Job drawing, mm, ordinate dimensions from the low corner. One solid piece. Round coordinates to 2 decimals unless told otherwise and drop trailing zeros. Order: outer loops, then holes, each group sorted by start corner. A loop starts at its lowest first (then second) coordinate and runs counter-clockwise, first axis right, second up. Notation, with made-up numbers: (73, -6.75) -> (104, -6.75) arc R19 ccw to (104, 26.25) -> close; hole circle Ø11 at (-31.75, 38). An arc over 180 degrees is marked (long way). Answer as a JSON object with one key per item and string values. Group by question number.
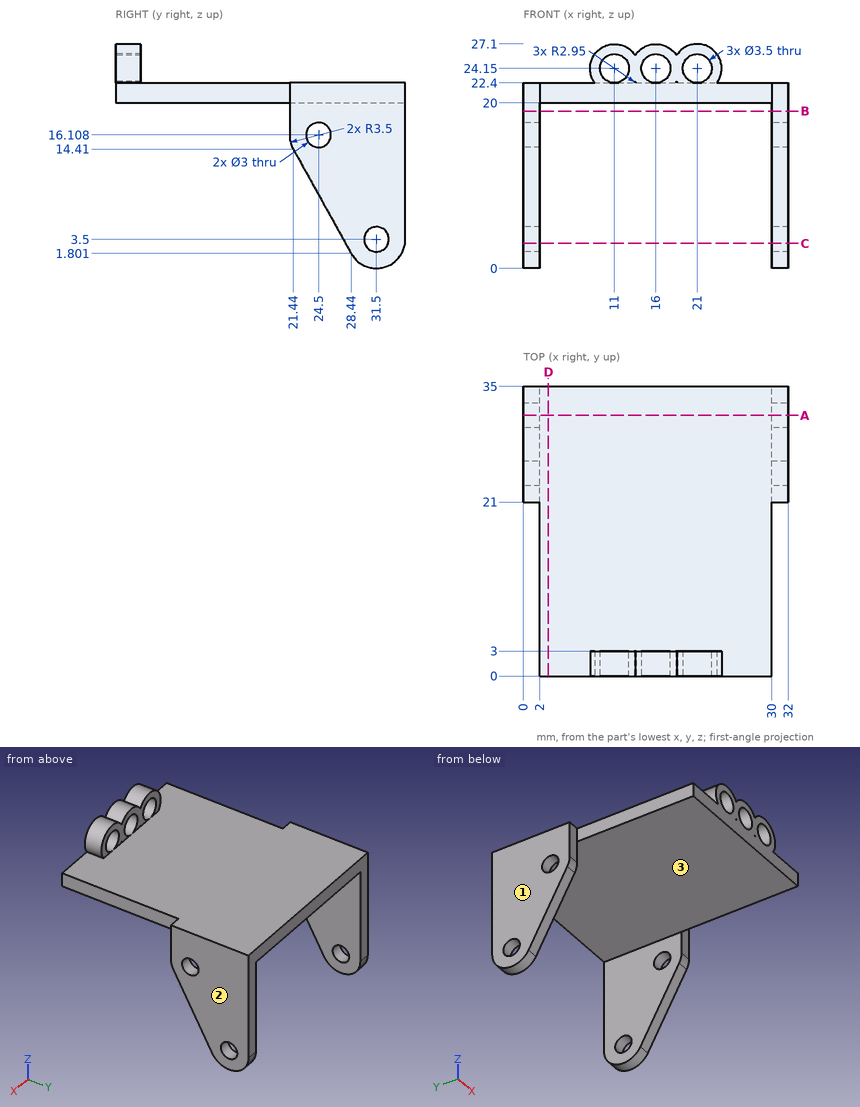
Q1. Band-saw the part on A-A (y = 31.5). List the corners of the cut face in (x, z), plus the area to 3 significant figures.
Q2. Wall check: line 1 (X direction, y = 1.05, z = 24.15); line 2 (Z direction, x = 16, y = 1.5); line 3 (X direction, y = 29.5, z = 8). Give the ranges that are in metal, low to high. Write a range as [from, to].
Q3. Band-saw the part on D-D (x = 3). List the corners of the cut face in (y, z).
Q4. Band-saw the part on B-B (z = 19). List the corners of the cut face in (x, y).
Q5. Band-saw the part on C-C (z = 3). List the corners of the cut face in (x, y) (1 decimal).
Q6. Drop flat-ended pins along their axis: pin 1 Ø12 at (x, y) = (9.5, 14) entering from -Z; pin 2 Ø4 at (x, z) = (15, 24.5) entering from +Y; pin 3 Ø0.7 at (y, z) = (7, 22) entering from +X; pin 4 Ø2.5 at (y, z) = (31.5, 3.5) entering from +X. Give the stop position or say it passes through.
Q7. Two-plate mould, pull along X, no slides. Class the marked faces 1, 2 and 3: +X half, -X half, draft (parallel to the pull), parting line (faces both ways), or undercut.
Completed:
{
 "1": {"outline": "(0, 0) -> (2, 0) -> (2, 2) -> (0, 2) -> close; (0, 5) -> (2, 5) -> (2, 20) -> (30, 20) -> (30, 5) -> (32, 5) -> (32, 22.4) -> (0, 22.4) -> close; (30, 0) -> (32, 0) -> (32, 2) -> (30, 2) -> close", "area": "145 mm2"},
 "2": {"line 1": "[8.05, 9.25], [12.75, 14.25], [17.75, 19.25], [22.75, 23.95]", "line 2": "[20, 22.4], [25.9, 27.1]", "line 3": "[0, 2], [30, 32]"},
 "3": {"outline": "(0, 20) -> (35, 20) -> (35, 22.4) -> (0, 22.4) -> close"},
 "4": {"outline": "(0, 21) -> (2, 21) -> (2, 35) -> (0, 35) -> close; (30, 21) -> (32, 21) -> (32, 35) -> (30, 35) -> close"},
 "5": {"outline": "(0, 27.8) -> (2, 27.8) -> (2, 30.1) -> (0, 30.1) -> close; (0, 32.9) -> (2, 32.9) -> (2, 35) -> (0, 35) -> close; (30, 27.8) -> (32, 27.8) -> (32, 30.1) -> (30, 30.1) -> close; (30, 32.9) -> (32, 32.9) -> (32, 35) -> (30, 35) -> close"},
 "6": {"pin 1": "z = 20", "pin 2": "y = 3", "pin 3": "x = 30", "pin 4": "through"},
 "7": {"face 1": "-X half", "face 2": "+X half", "face 3": "undercut"}
}
